Can you work these out from the model? Positions are in its coordinate system, mm. A direction names the side the tool comes from. Coordinates: 2 decimals unless noted, no trailing zeros. Order: outer loops, then holes, each group sorted by start corner. A loop starts at its lowest first (then second) coordinate and runs counter-clockwise, first axis right, second up. Notation, with made-up numbers: (52, -7.75) -> (108, -7.75) arc R9 cw to (108, 1.25) -> close; hole circle Ø6 at (-22.5, 42). An arc over 180 degrees is marked (long way). Return JSON: item names as keys, results as strings. Group by question number.
1) Thinking about a two-plate mould opening in Z: for faces 1 (the flat face through (-9, 43.8, 0)), 2 (the flat face through (0, 51, -4)), 3 (the flat face through (9, 43.8, 0)), 4 (the flat face through (0, 44, 7.2)), which applies, +Z half, -Z half, draft (parallel to the pull), parting line (faces both ways), or undercut?
2) If I drill on probe 1 along Y at (x, z) = (-2, -7.25); probe 2 along Z at (x, y) = (-6.25, 44.25); probe 3 along X at (y, z) = (47.25, 0), over which ranges is the centre line in solid material (lowest first)? Write a range as from..to.
3) For faces 5 (the flat face through (0, 43.5, 0)), 6 (the cylindrical face through (9.41, 44.49, -1.91)), 7 (the cylindrical face through (0, 51, 5)), 8 (the flat face through (3.7, 49, -8)), 9 (the flat face through (0, 44, -7.2)), which set-ups out of +Z, -Z, +X, -X, +Y, -Y let a thin tool reach every point of the face, with its end or its side?
4) For pin 1 (1.4 mm diameter, centred on x = 8.5, z = 0.5, fed in from +Y); pin 2 (1.6 mm diameter, centred on x = -3, y = 44.5, fed in from -Z); pin 3 (1 mm diameter, centred on y = 48.5, z = -6.5, fed in from +X), each with a flat end and sliding along its axis, tell me the tip position at first contact or that it passes through.
5) If we section it at A-A, the plane y = 47: Please give me the cut outline in (x, z).
6) If we section it at B-B, the plane x = 0: Please give me the cut outline in (y, z).
7) If we section it at C-C, the plane z = 0: Please give me the cut outline in (x, y), then the cut area to 3 significant figures.
from build123d import *

# Parameters (mm, degrees)
PAD037_DEPTH    = 2
PAD043_DEPTH    = 5
PAD018_DEPTH    = 2
SKETCH069_R     = 1.6
POCKET020_DEPTH = 6.7
SKETCH071_W     = 7.4
SKETCH071_H     = 2
PAD045_DEPTH    = 1.5


with BuildPart() as part:
    # Sketch051 → Pad037 (new body)
    with BuildSketch(Plane.XZ.offset(-17.8)):
        with BuildLine():
            ThreePointArc((-6.3498031466, 7.2), (-9.6, 0), (-6.3498031466, -7.2))
            Line((-6.3498031466, -7.2), (6.3498031466, -7.2))
            ThreePointArc((6.3498031466, -7.2), (9.6, 0), (6.3498031466, 7.2))
            Line((-6.3498031466, 7.2), (6.3498031466, 7.2))
        make_face()
    extrude(amount=-PAD037_DEPTH)

    # Sketch067 (on Face6 of Pad037) → Pad043 (join)
    with BuildSketch(Plane(origin=(0, 19.8, 0), x_dir=(1, 0, 0), z_dir=(0, 1, 0))):
        with BuildLine():
            ThreePointArc((-6.4621977686, 7.5), (-9.9, 0), (-6.4621977686, -7.5))
            Line((-6.4621977686, -7.5), (6.4621977686, -7.5))
            ThreePointArc((6.4621977686, -7.5), (9.9, 0), (6.4621977686, 7.5))
            Line((-6.4621977686, 7.5), (6.4621977686, 7.5))
        make_face()
    extrude(amount=PAD043_DEPTH)

    # Sketch068 (on Face5 of Pad043) → Pad018 (join)
    with BuildSketch(Plane(origin=(0, 24.8, 0), x_dir=(1, 0, 0), z_dir=(0, 1, 0))):
        with BuildLine():
            ThreePointArc((-3, 4), (0, -5), (3, 4))
            Line((-3, 4), (3, 4))
        make_face()
    extrude(amount=PAD018_DEPTH)

    # Sketch069 (on Face5 of Pad018) → Pocket020 (cut)
    with BuildSketch(Plane(origin=(0, 24.8, 0), x_dir=(1, 0, 0), z_dir=(0, 1, 0))):
        with Locations((-9.5, 0)):
            Circle(SKETCH069_R)
        with Locations((9.5, 0)):
            Circle(SKETCH069_R)
    extrude(amount=-POCKET020_DEPTH, mode=Mode.SUBTRACT)

    # Sketch071 (on Face4 of Pocket020) → Pad045 (join)
    with BuildSketch(Plane(origin=(0, 0, -7.5), x_dir=(1, 0, 0), z_dir=(0, 0, -1))):
        with Locations((0, -23.8)):
            Rectangle(SKETCH071_W, SKETCH071_H)
    extrude(amount=PAD045_DEPTH)

    # Sketch072 → Groove (revolve, cut)
    with BuildSketch(Plane.XY):
        with BuildLine():
            ThreePointArc((-7.4, 24.8), (-9.167766953, 24.067766953), (-9.9, 22.3))
            Line((-9.9, 24.8), (-9.9, 22.3))
            Line((-9.9, 24.8), (-7.4, 24.8))
        make_face()
    revolve(axis=Axis((0, 0, 0), (0, 1, 0)), mode=Mode.SUBTRACT)


with BuildPart() as part_1:
    # Body023 placement: moved
    add(part.part.moved(Location((0, 25.7, 0))))


solid = part_1.part
Result sheet:
{
 "1": {"face 1": "undercut", "face 2": "-Z half", "face 3": "undercut", "face 4": "+Z half"},
 "2": {"probe 1": "y = 45.5..50.5", "probe 2": "z = -7.2..7.2", "probe 3": "x = -7.9..7.9"},
 "3": {"face 5": "+Z, -Z, +X, -X, -Y", "face 6": "+X, -Y", "face 7": "+Y", "face 8": "-Z, +X, +Y, -Y", "face 9": "-Z, +X, -X, -Y"},
 "4": {"pin 1": "stops at y = 50.47", "pin 2": "stops at z = -7.2", "pin 3": "stops at x = 7.83"},
 "5": {"outline": "(-9.77, -1.58) arc R9.9 ccw to (-6.46, -7.5) -> (6.46, -7.5) arc R9.9 ccw to (9.77, -1.58) arc R1.6 cw (long way) to (9.77, 1.58) arc R9.9 ccw to (6.46, 7.5) -> (-6.46, 7.5) arc R9.9 ccw to (-9.77, 1.58) arc R1.6 cw (long way) to start"},
 "6": {"outline": "(43.5, -7.2) -> (45.5, -7.2) -> (45.5, -7.5) -> (48.5, -7.5) -> (48.5, -9) -> (49.92, -9) arc R2.5 ccw to (50.5, -7.4) -> (50.5, -4) -> (52.5, -4) -> (52.5, 5) -> (50.5, 5) -> (50.5, 7.4) arc R2.5 ccw to (50.5, 7.5) -> (45.5, 7.5) -> (45.5, 7.2) -> (43.5, 7.2) -> close"},
 "7": {"outline": "(-9.6, 43.5) -> (9.6, 43.5) -> (9.6, 43.8) -> (7.9, 43.8) -> (7.9, 50.45) arc R2.5 ccw to (7.4, 50.5) -> (5, 50.5) -> (5, 52.5) -> (-5, 52.5) -> (-5, 50.5) -> (-7.4, 50.5) arc R2.5 ccw to (-7.9, 50.45) -> (-7.9, 43.8) -> (-9.6, 43.8) -> close", "area": "132 mm2"}
}
